Verification items for the finished model (mm, model axes). A direction names the side the tool comes from. Round coordinates to 2 decimals unless told otherwise and drop trailing zeros. Order: outer loops, then holes, each group sorted by start corner. A loop starts at its lowest first (then second) coordinate and runs counter-clockwise, first axis right, second up. Notation, with made-up numbers: (70, 15) -> (125, 15) arc R17 cw to (125, 33) -> close; hole circle Ø9 at (-38, 62). An arc over 180 degrees is marked (long way). Answer in a Markdown table with one row per item. Add a question column.
```python
from build123d import *

# Parameters (mm, degrees)
BOSS_EXTRUDE1_DEPTH = 10
FILLET1_R           = 5
CUT_EXTRUDE3_START  = -2
SKETCH3_R           = 2
CUT_EXTRUDE3_DEPTH  = 8


with BuildPart() as part:
    # Sketch1 → Boss-Extrude1 (new body)
    with BuildSketch(Plane(origin=(0, 0, 0), x_dir=(1, 0, 0), z_dir=(0, 1, 0))):
        with BuildLine():
            Line((115.149446157, 11.244299939), (107.390918627, -18.755700061))
            ThreePointArc((107.390918627, -18.755700061), (102.051963222, -26.860343606), (92.868704021, -30))
            Line((92.868704021, -30), (-92.868704021, -30))
            ThreePointArc((-92.868704021, -30), (-102.051963222, -26.860343606), (-107.390918627, -18.755700061))
            Line((-107.390918627, -18.755700061), (-115.149446157, 11.244299939))
            ThreePointArc((-115.149446157, 11.244299939), (-112.487575158, 24.183259201), (-100.627231552, 30))
            Line((-100.627231552, 30), (100.627231552, 30))
            ThreePointArc((100.627231552, 30), (112.487575158, 24.183259201), (115.149446157, 11.244299939))
        make_face()
    extrude(amount=BOSS_EXTRUDE1_DEPTH)

    # Fillet1
    fillet1_edges = [part.edges().sort_by_distance(p)[0] for p in [
        (0, 0, 30),
        (-102.051963222, 0, 26.860343606),
        (-111.270182392, 0, 3.755700061),
        (-112.487575158, 0, -24.183259201),
        (0, 10, 30),
        (102.051963222, 10, 26.860343606),
        (111.270182392, 10, 3.755700061),
        (112.487575158, 10, -24.183259201),
        (0, 10, -30),
        (0, 0, -30),
        (-111.270182392, 10, 3.755700061),
        (111.270182392, 0, 3.755700061),
    ]]
    fillet(fillet1_edges, radius=FILLET1_R - 0.0001)  # a hair under: the kernel refuses the full size

    # Sketch3 → Cut-Extrude3 (cut)
    with BuildSketch(Plane.XZ.offset(CUT_EXTRUDE3_START)):
        with Locations(Location((-70, 8, 0), (0, 0, 270))):
            Circle(SKETCH3_R)
        with Locations(Location((-70, -8, 0), (0, 0, 90))):
            Circle(SKETCH3_R)
        with Locations(Location((70, -8, 0), (0, 0, 270))):
            Circle(SKETCH3_R)
        with Locations(Location((70, 8, 0), (0, 0, 90))):
            Circle(SKETCH3_R)
    extrude(amount=-CUT_EXTRUDE3_DEPTH, mode=Mode.SUBTRACT)


solid = part.part
```
1) Thickness scan on L1, parallel to X at y = 5.5, z = 8; L2, parallel to X at y = 7.5, z = -8; L3, parallel to Z at x = -93.5, y = 5.5. Record the ranges inside material, lowest first. Write a range as [from, to].
2) Cross-section at A-A, the plane y = 8. Record the boundary of the cut face in (x, z), and give its area (3 significant figures).
3) Draft check along Z on faces 3 (the face through (-68, 6, 8)), 4 (the face through (1, 8, -29)), 5 (the face through (-70, 2, 8)), 6 (the face through (2, 10, 0)). Enter one of: +Z half, -Z half, draft (parallel to the pull), parting line (faces both ways), or undercut.
4) Depth check by flat-ended pin: P1, Ø2.5, axis at x = -70, z = -8, coming from the +Y side; P2, Ø5, axis at y = 1.5, z = 9.5, coming from the +X side; P3, Ø5, axis at y = 1.5, z = 11, coming from the -X side. Enter the tip coordinate at first touch or a pass-through.
5) Tool access check on faces 1 (the face through (-70, 2, -8)), 2 (the face through (109.836, 1.504, 3.609)). Record the directions out of +Z, -Z, +X, -X, +Y, -Y that give a thin tool (end or side, any length) a straight path to the whole face; none if there is none.
Results below:
| question | item | result |
|---|---|---|
| 1 | L1 | [-110.15, -72], [-68, 68], [72, 110.15] |
| 1 | L2 | [-113.62, -72], [-68, 68], [72, 113.62] |
| 1 | L3 | [-29.97, 29.96] |
| 2 | outline | (-114.18, -11.49) arc R14 ccw to (-100.63, -29) -> (100.63, -29) arc R14 ccw to (114.18, -11.49) -> (106.42, 18.51) arc R14 ccw to (92.87, 29) -> (-92.87, 29) arc R14 ccw to (-106.42, 18.51) -> close; hole circle Ø4 at (-70, -8); hole circle Ø4 at (-70, 8); hole circle Ø4 at (70, -8); hole circle Ø4 at (70, 8) |
| 2 | area | 12,700 mm² |
| 3 | face 3 | undercut |
| 3 | face 4 | -Z half |
| 3 | face 5 | undercut |
| 3 | face 6 | draft |
| 4 | P1 | y = 2 |
| 4 | P2 | x = 109.93 |
| 4 | P3 | x = -109.55 |
| 5 | face 1 | +Y |
| 5 | face 2 | +Z, +X, -Y |
